CAD build for the part. Positions are in the model's coordinates, mm. Face numbers are marked on the shaded views. A direction names the side the tool comes from. Round coordinates to 2 decimals unless told otherwise and drop trailing zeros. Loops run counter-clockwise (first coordinate to the right, second up) from the corner with the lowest first, then second, coordinate; pieces in that order, holes last. Notation, with made-up numbers: M 49.25,-21.5 L 81.25,-21.5 A37 ccw 81.25,16.5 Z; hole C 42.5,58 d9. An arc over 180 degrees is marked long. Use a Markdown table: item, result. Add a question column.
(1) Wall check: L1, parallel to Z at x = 3, y = 0; L2, parallel to Z at x = 2.5, y = 0.5; L3, parallel to Y at x = -1.25, z = 0.5. Give the ranges that are in metal, low to high.
(2) Band-saw the part on B-B, the plane x = 0. Write the cut outline in (y, z).
(3) Band-saw the part on A-A, the plane z = 9. Write the cut outline in (x, y).
(4) Flat gauge pin, fed straight in: P1, Ø2, axis at y = 0.5, z = 10, coming from the +X side. Where does the tip first touch, or does it go through?
(5) Which spindle directions (+Z, -Z, +X, -X, +Y, -Y) get a long thin tool onto all of the face, cutting with end or side? Do the marked faces 1 and 2. Say none if no direction does.
from build123d import *

# Parameters (mm, degrees)
BOSS_EXTRUDE6_DEPTH  = 1.5
SKETCH4_R            = 2.6
BOSS_EXTRUDE7_DEPTH  = 0.3
SKETCH5_R            = 2.4
BOSS_EXTRUDE10_DEPTH = 12
CHAMFER3_SIZE        = 0.4


with BuildPart() as part:
    # Sketch2 → Boss-Extrude6 (new body)
    with BuildSketch(Plane.XY):
        Polygon((1.792912768, 3.012681291), (-1.712602147, 3.05904865), (-3.505514916, 0.046367359), (-1.792912768, -3.012681291), (1.712602147, -3.05904865), (3.505514916, -0.046367359), align=None)
    extrude(amount=BOSS_EXTRUDE6_DEPTH)

    # Sketch4 → Boss-Extrude7 (add)
    with BuildSketch(Plane.XY.offset(1.5)):
        Circle(SKETCH4_R)
    extrude(amount=BOSS_EXTRUDE7_DEPTH)

    # Sketch5 → Boss-Extrude10 (add)
    with BuildSketch(Plane.XY.offset(1.8)):
        Circle(SKETCH5_R)
    extrude(amount=BOSS_EXTRUDE10_DEPTH)

    # Chamfer3
    chamfer3_edges = [part.edges().sort_by_distance(p)[0] for p in [
        (-2.4, 0, 13.8),
    ]]
    chamfer(chamfer3_edges, length=CHAMFER3_SIZE)


solid = part.part
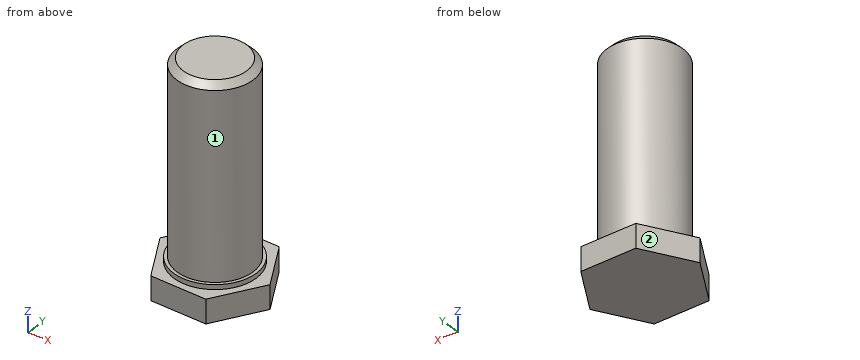
Return value:
| question | item | result |
|---|---|---|
| 1 | L1 | 0 to 1.5 |
| 1 | L2 | 0 to 1.8 |
| 1 | L3 | -3.02 to 3.05 |
| 2 | outline | M -3.04,0 L 3.04,0 L 3.04,1.5 L 2.6,1.5 L 2.6,1.8 L 2.4,1.8 L 2.4,13.4 L 2,13.8 L -2,13.8 L -2.4,13.4 L -2.4,1.8 L -2.6,1.8 L -2.6,1.5 L -3.04,1.5 Z |
| 3 | outline | C 0,0 d4.8 |
| 4 | P1 | x = 2.4 |
| 5 | face 1 | +Z |
| 5 | face 2 | +Z, -Z, -X, +Y |
